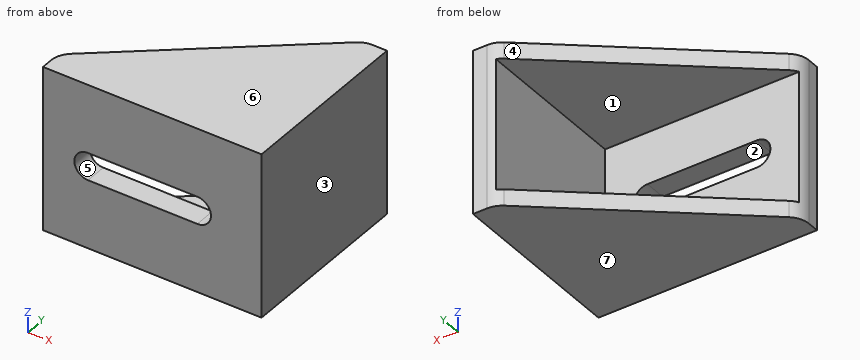
```python
from build123d import *

# Parameters (mm, degrees)
BOSS_EXTRUDE1_DEPTH = 38.1
BOSS_EXTRUDE2_DEPTH = 3.81
FILLET3_START       = -1
FILLET3_DEPTH       = 40
CUT_EXTRUDE1_REACH  = 75.408


with BuildPart() as part:
    # Sketch1 → Boss-Extrude1 (new body)
    with BuildSketch(Plane.XY):
        Polygon((-50.8, 0), (0, 0), (0, 41.91), (-5.08, 41.91), (-5.08, 5.08), (-50.8, 5.08), align=None)
    extrude(amount=BOSS_EXTRUDE1_DEPTH)

    # Sketch6 → Boss-Extrude2 (add)
    with BuildSketch(Plane.XY):
        Polygon((-50.8, 5.08), (-5.08, 5.08), (-5.08, 41.91), align=None)
    boss_extrude2 = extrude(amount=BOSS_EXTRUDE2_DEPTH)

    # Mirror1: Boss-Extrude2 across plane
    add(boss_extrude2.mirror(Plane.XY.offset(19.05)))

    # Fillet3: read off the stored shape, not the designer's step
    # Fillet3 outline → Fillet3 (cut)
    with BuildSketch(Plane.XY.offset(FILLET3_START)):
        with BuildLine():
            Line((-48.906834052, 6.605050347), (-50.8, 5.08))
            Line((-50.8, 5.08), (-50.8, 2.648980489))
            ThreePointArc((-50.8, 2.648980489), (-50.30233112, 4.841841977), (-48.906834052, 6.605050347))
        make_face()
        with BuildLine():
            Line((-5.08, 41.91), (-6.475223624, 40.786069858))
            ThreePointArc((-6.475223624, 40.786069858), (-4.977999752, 41.620784637), (-3.288389572, 41.91))
            Line((-3.288389572, 41.91), (-5.08, 41.91))
        make_face()
    extrude(amount=FILLET3_DEPTH, mode=Mode.SUBTRACT)

    # Sketch2 → Cut-Extrude1 (cut, up to next)
    with BuildSketch(Plane(origin=(0, 5.08, 0), x_dir=(1, 0, 0), z_dir=(0, 1, 0)), mode=Mode.PRIVATE) as cut_extrude1_sk1:
        with BuildLine():
            Line((-40.33027712, -15.875), (-14.93027712, -15.875))
            ThreePointArc((-14.93027712, -15.875), (-11.75527712, -19.05), (-14.93027712, -22.225))
            Line((-14.93027712, -22.225), (-40.33027712, -22.225))
            ThreePointArc((-40.33027712, -22.225), (-43.50527712, -19.05), (-40.33027712, -15.875))
        make_face()
    cut_extrude1_tool1 = extrude(cut_extrude1_sk1.sketch, amount=-CUT_EXTRUDE1_REACH, mode=Mode.PRIVATE) & part.part
    add(cut_extrude1_tool1.solids().sort_by_distance((-27.630277, 5.08, 19.05))[0], mode=Mode.SUBTRACT)


solid = part.part
```
Model file for the job. Use its own axes, mm. Face numbers are marked on the shaded views. A direction names the side the tool comes from. Coordinates: 2 decimals unless noted, no trailing zeros. Loops run counter-clockwise (first coordinate to the right, second up) from the corner with the lowest first, then second, coordinate; pieces in that order, holes last. Notation, with made-up numbers: (19, -0.75) - (40, -0.75) arc R19 cw to (40, 32.25) - close; hole circle Ø8 at (29, 31.25). An arc over 180 degrees is marked (long way). Write item = value, one per line. Start each with the question number.
Item 1: Saw through at A-A, the plane z = 19.05. List the corners of the cut face in (x, y), then the cut area to 3 significant figures.
Item 2: Pull direction Z, two halves, no side cores. Call the marked faces 4, 5, 6 and 7: +Z half, -Z half, draft (parallel to the pull), parting line (faces both ways), or undercut.
Item 3: 3-axis set-ups, long thin cutter, end or side, ignore diameter. For the marked faces 1, 2 and 3: which of +Z, -Z, +X, -X, +Y, -Y reach the whole face in a straight line?
Item 4: Drop flat-ended pins along their axis: pin 1 Ø3 at (y, z) = (32, 24.5) entering from -X; pin 2 Ø2 at (x, y) = (-26.5, 28.5) entering from -Z. Give the stop position or say it passes through.
Item 5: Wall check: probe 1 along Z at (x, y) = (-10, 22.5); probe 2 along Z at (x, y) = (-40, 5) (3 decimals); probe 3 along X at (y, z) = (23, 15). Give the ranges that are in metal, low to high. Write a range as [from, to].
Item 6: Saw through at D-D, the plane y = 4. List the corners of the cut face in (x, z) (3 decimals), then the cut area to 3 significant figures.
Item 7: Saw through at B-B, the plane x = -17. List the corners of the cut face in (y, z) (3 decimals), then the cut area to 3 significant figures.
Item 8: Saw through at C-C, the plane z = 36.5. List the corners of the cut face in (x, y), then the cut area to 3 significant figures.
Answers:
q1.outline = (-50.8, 0) - (-43.51, 0) - (-43.51, 5.08) - (-50.18, 5.08) arc R5.08 ccw to (-50.8, 2.65) - close; (-11.76, 0) - (0, 0) - (0, 41.91) - (-3.29, 41.91) arc R5.08 ccw to (-5.08, 41.58) - (-5.08, 5.08) - (-11.76, 5.08) - close
q1.area = 283 mm2
q2.face_4 = draft
q2.face_5 = undercut
q2.face_6 = +Z half
q2.face_7 = -Z half
q3.face_1 = -X, +Y
q3.face_2 = +Y, -Y
q3.face_3 = +Z, -Z, +X, +Y, -Y
q4.pin_1 = -5.08
q4.pin_2 = through
q5.probe_1 = [0, 3.81], [34.29, 38.1]
q5.probe_2 = [0, 15.875], [22.225, 38.1]
q5.probe_3 = [-5.08, 0]
q6.outline = (-50.617, 0) - (0, 0) - (0, 38.1) - (-50.617, 38.1) - close; hole (-40.33, 15.875) - (-14.93, 15.875) arc R3.175 ccw to (-14.93, 22.225) - (-40.33, 22.225) arc R3.175 ccw to start
q6.area = 1,740 mm2
q7.outline = (0, 0) - (32.308, 0) - (32.308, 3.81) - (5.08, 3.81) - (5.08, 15.875) - (0, 15.875) - close; (0, 22.225) - (5.08, 22.225) - (5.08, 34.29) - (32.308, 34.29) - (32.308, 38.1) - (0, 38.1) - close
q7.area = 369 mm2
q8.outline = (-50.8, 0) - (0, 0) - (0, 41.91) - (-3.29, 41.91) arc R5.08 ccw to (-6.48, 40.79) - (-48.91, 6.61) arc R5.08 ccw to (-50.8, 2.65) - close
q8.area = 1,290 mm2
